Check sheet for the modelled part. Datum: model origin and axes. Units: mm. A direction names the side the tool comes from. Give positions to 0.01 mm unless a question says otherwise; leave off trailing zeros. Loops run counter-clockwise (first coordinate to the right, second up) from the corner with the lowest first, then second, coordinate; pieces in that order, holes last. Notation, with made-up numbers: (14.25, -16) - (22.25, -16) arc R11 ccw to (22.25, -6) - close; hole circle Ø1 at (-26.75, 47). An arc over 180 degrees is marked (long way). Use one line per item in the form item = value.
from build123d import *

# Parameters (mm, degrees)
SKETCH1_R                                    = 34
SKETCH1_R_2                                  = 20
OUTPUT_PLATE_DEPTH                           = 4
Y_TONGUE_1_START                             = 3.99
SKETCH2_W                                    = 4
SKETCH2_H                                    = 10
Y_TONGUE_1_DEPTH                             = 2.01
SKETCH3_W                                    = 4
SKETCH3_H                                    = 10
Y_TONGUE_1_2_DEPTH                           = 2.01
SKETCH4_R                                    = 1.1
FOUR_M2_CLEARANCE_DEPTH                      = 4.01
SKETCH5_R                                    = 2.1
FOUR_90DEG_COUNTERSINKS_D4P2_DEPTH           = 1.1
FOUR_90DEG_COUNTERSINKS_D4P2_DRAFT           = -45
FOUR_90DEG_COUNTERSINKS_D4P2_PROFILE_2_DEPTH = 1.1
FOUR_90DEG_COUNTERSINKS_D4P2_PROFILE_2_DRAFT = -45
FOUR_90DEG_COUNTERSINKS_D4P2_PROFILE_3_DEPTH = 1.1
FOUR_90DEG_COUNTERSINKS_D4P2_PROFILE_3_DRAFT = -45
FOUR_90DEG_COUNTERSINKS_D4P2_PROFILE_4_DEPTH = 1.1
FOUR_90DEG_COUNTERSINKS_D4P2_PROFILE_4_DRAFT = -45
SKETCH6_R                                    = 1.51
FOUR_STANDOFF_PILOT_POCKETS_D3P02_DEPTH      = 1.1


with BuildPart() as part:
    # Sketch1 → Output_Plate (new body)
    with BuildSketch(Plane.XY):
        Circle(SKETCH1_R)
        Circle(SKETCH1_R_2, mode=Mode.SUBTRACT)
    extrude(amount=OUTPUT_PLATE_DEPTH)

    # Sketch2 → Y_Tongue_-1 (add)
    with BuildSketch(Plane.XY.offset(Y_TONGUE_1_START)):
        with Locations((0, -33)):
            Rectangle(SKETCH2_W, SKETCH2_H)
    extrude(amount=Y_TONGUE_1_DEPTH)

    # Sketch3 → Y_Tongue_1 2 (add)
    with BuildSketch(Plane.XY.offset(Y_TONGUE_1_START)):
        with Locations((0, 33)):
            Rectangle(SKETCH3_W, SKETCH3_H)
    extrude(amount=Y_TONGUE_1_2_DEPTH)

    # Sketch4 → Four_M2_Clearance (cut)
    with BuildSketch(Plane.XY.offset(4)):
        with Locations((27.716385975, 11.480502971)):
            Circle(SKETCH4_R)
        with Locations((-11.480502971, 27.716385975)):
            Circle(SKETCH4_R)
        with Locations((-27.716385975, -11.480502971)):
            Circle(SKETCH4_R)
        with Locations((11.480502971, -27.716385975)):
            Circle(SKETCH4_R)
    extrude(amount=-FOUR_M2_CLEARANCE_DEPTH, mode=Mode.SUBTRACT)


with BuildPart() as four_90deg_countersinks_d4p2_tool:
    # Sketch5 → Four_90deg_Countersinks_D4p2 (with draft: the straight prism first)
    with BuildSketch(Plane.XY.offset(4)):
        with Locations((27.716385975, 11.480502971)):
            Circle(SKETCH5_R)
    extrude(amount=-FOUR_90DEG_COUNTERSINKS_D4P2_DEPTH)
    # Four_90deg_Countersinks_D4p2: the draft: its side faces are tilted about the plane it starts from
    four_90deg_countersinks_d4p2_sides = [four_90deg_countersinks_d4p2_tool.faces().sort_by_distance(p)[0] for p in [
        (25.616385975, 11.480502971, 3.45),
    ]]
    draft(four_90deg_countersinks_d4p2_sides, Plane.XY.offset(4), FOUR_90DEG_COUNTERSINKS_D4P2_DRAFT)


with BuildPart() as part_1:
    add(part.part)

    # Four_90deg_Countersinks_D4p2: cut by four_90deg_countersinks_d4p2_tool
    add(four_90deg_countersinks_d4p2_tool.part, mode=Mode.SUBTRACT)


with BuildPart() as four_90deg_countersinks_d4p2_profile_2_tool:
    # Sketch5 → Four_90deg_Countersinks_D4p2 profile 2 (with draft: the straight prism first)
    with BuildSketch(Plane.XY.offset(4)):
        with Locations((-11.480502971, 27.716385975)):
            Circle(SKETCH5_R)
    extrude(amount=-FOUR_90DEG_COUNTERSINKS_D4P2_PROFILE_2_DEPTH)
    # Four_90deg_Countersinks_D4p2 profile 2: the draft: its side faces are tilted about the plane it starts from
    four_90deg_countersinks_d4p2_profile_2_sides = [four_90deg_countersinks_d4p2_profile_2_tool.faces().sort_by_distance(p)[0] for p in [
        (-13.580502971, 27.716385975, 3.45),
    ]]
    draft(four_90deg_countersinks_d4p2_profile_2_sides, Plane.XY.offset(4), FOUR_90DEG_COUNTERSINKS_D4P2_PROFILE_2_DRAFT)


with BuildPart() as part_2:
    add(part_1.part)

    # Four_90deg_Countersinks_D4p2 profile 2: cut by four_90deg_countersinks_d4p2_profile_2_tool
    add(four_90deg_countersinks_d4p2_profile_2_tool.part, mode=Mode.SUBTRACT)


with BuildPart() as four_90deg_countersinks_d4p2_profile_3_tool:
    # Sketch5 → Four_90deg_Countersinks_D4p2 profile 3 (with draft: the straight prism first)
    with BuildSketch(Plane.XY.offset(4)):
        with Locations((-27.716385975, -11.480502971)):
            Circle(SKETCH5_R)
    extrude(amount=-FOUR_90DEG_COUNTERSINKS_D4P2_PROFILE_3_DEPTH)
    # Four_90deg_Countersinks_D4p2 profile 3: the draft: its side faces are tilted about the plane it starts from
    four_90deg_countersinks_d4p2_profile_3_sides = [four_90deg_countersinks_d4p2_profile_3_tool.faces().sort_by_distance(p)[0] for p in [
        (-29.816385975, -11.480502971, 3.45),
    ]]
    draft(four_90deg_countersinks_d4p2_profile_3_sides, Plane.XY.offset(4), FOUR_90DEG_COUNTERSINKS_D4P2_PROFILE_3_DRAFT)


with BuildPart() as part_3:
    add(part_2.part)

    # Four_90deg_Countersinks_D4p2 profile 3: cut by four_90deg_countersinks_d4p2_profile_3_tool
    add(four_90deg_countersinks_d4p2_profile_3_tool.part, mode=Mode.SUBTRACT)


with BuildPart() as four_90deg_countersinks_d4p2_profile_4_tool:
    # Sketch5 → Four_90deg_Countersinks_D4p2 profile 4 (with draft: the straight prism first)
    with BuildSketch(Plane.XY.offset(4)):
        with Locations((11.480502971, -27.716385975)):
            Circle(SKETCH5_R)
    extrude(amount=-FOUR_90DEG_COUNTERSINKS_D4P2_PROFILE_4_DEPTH)
    # Four_90deg_Countersinks_D4p2 profile 4: the draft: its side faces are tilted about the plane it starts from
    four_90deg_countersinks_d4p2_profile_4_sides = [four_90deg_countersinks_d4p2_profile_4_tool.faces().sort_by_distance(p)[0] for p in [
        (9.380502971, -27.716385975, 3.45),
    ]]
    draft(four_90deg_countersinks_d4p2_profile_4_sides, Plane.XY.offset(4), FOUR_90DEG_COUNTERSINKS_D4P2_PROFILE_4_DRAFT)


with BuildPart() as part_4:
    add(part_3.part)

    # Four_90deg_Countersinks_D4p2 profile 4: cut by four_90deg_countersinks_d4p2_profile_4_tool
    add(four_90deg_countersinks_d4p2_profile_4_tool.part, mode=Mode.SUBTRACT)

    # Sketch6 → Four_Standoff_Pilot_Pockets_D3p02 (cut)
    with BuildSketch(Plane(origin=(0, 0, 0), x_dir=(-1, 0, 0), z_dir=(0, 0, -1))):
        with Locations((-27.716385975, 11.480502971)):
            Circle(SKETCH6_R)
        with Locations((11.480502971, 27.716385975)):
            Circle(SKETCH6_R)
        with Locations((27.716385975, -11.480502971)):
            Circle(SKETCH6_R)
        with Locations((-11.480502971, -27.716385975)):
            Circle(SKETCH6_R)
    extrude(amount=-FOUR_STANDOFF_PILOT_POCKETS_D3P02_DEPTH, mode=Mode.SUBTRACT)


solid = part_4.part
Item 1: Thickness scan on L1, parallel to Y at x = 0, z = 1.5; L2, parallel to X at y = -11, z = 1.75; L3, parallel to Y at x = 11.5, z = 1.6. Record the ranges inside material, lowest first.
Answer block:
L1 = -34 to -20, 20 to 34
L2 = -32.17 to -28.71, -26.73 to -16.7, 16.7 to 32.17
L3 = -32 to -28.82, -26.62 to -16.36, 16.36 to 32
Item 2: Mould release check, pull along X, two halves, no side actions. Record for faces 1 (the face through (-11.624, 28.807, 2.063)), 2 (the face through (0, -36, 3.99)), 3 (the face through (-2, -33, 5)): released by +X, released by -X, zero draft, split by the parting line, or undercut.
Answer block:
face_1 = undercut
face_2 = zero draft
face_3 = released by -X
Item 3: Access from +Z, -Z, +X, -X, +Y, -Y to the whole of each face (thin tool, end or side, straight path). Record for faces 4 (the face through (0, 28, 5)), 5 (the face through (-29.157, -11.027, 0.542)), 6 (the face through (0, 33, 6)).
Answer block:
face_4 = +Z, +X, -X
face_5 = -Z
face_6 = +Z, +X, -X, +Y, -Y
Item 4: Section check A-A on y = -16. Record the boundary of the cut face in (x, z).
Answer block:
outline = (-30, 0) - (-12, 0) - (-12, 4) - (-30, 4) - close; (12, 0) - (30, 0) - (30, 4) - (12, 4) - close
Item 5: Gauge pin test, flat ends, axial feed: P1, Ø4, axis at x = 1.5, y = -18.5, coming from the +Z side; P2, Ø3, axis at x = 3.5, z = 1, coming from the +Y side; P3, Ø4, axis at x = 11.48, y = -27.72, coming from the +Z side; P4, Ø1.8, axis at x = -27.72, y = -11.48, coming from the -Z side (1 decimal). Record the tip position at first contact, or that the pin passes through.
Answer block:
P1 = 4
P2 = 33.94
P3 = 3.9
P4 = through
Item 6: Section check B-B on x = 0. Record the boundary of the cut face in (y, z), then the cut area to 3 significant figures.
Answer block:
outline = (-38, 3.99) - (-34, 3.99) - (-34, 0) - (-20, 0) - (-20, 4) - (-28, 4) - (-28, 6) - (-38, 6) - close; (20, 0) - (34, 0) - (34, 3.99) - (38, 3.99) - (38, 6) - (28, 6) - (28, 4) - (20, 4) - close
area = 152 mm2
Item 7: Section check D-D on y = 31. Record the boundary of the cut face in (x, z), then the cut area to 3 significant figures.
Answer block:
outline = (-13.96, 0) - (13.96, 0) - (13.96, 4) - (2, 4) - (2, 6) - (-2, 6) - (-2, 4) - (-13.96, 4) - close
area = 120 mm2
Item 8: Section check C-C on y = 0. Record the boundary of the cut face in (x, z).
Answer block:
outline = (-34, 0) - (-20, 0) - (-20, 4) - (-34, 4) - close; (20, 0) - (34, 0) - (34, 4) - (20, 4) - close
